For this review, take the finished solid that the model builds, in its own axes (mm). A direction names the side the tool comes from. Round coordinates to 2 decimals unless told otherwise and drop trailing zeros. Order: outer loops, then holes, each group sorted by start corner. A loop starts at its lowest first (then second) coordinate and runs counter-clockwise, first axis right, second up. Notation, with made-up numbers: M -18.5,77 L -0.5,77 A19 ccw -0.5,103 Z; hole C 39,-20.5 d9. An arc over 180 degrees is marked long. Use a Markdown table: item, result.
from build123d import *

# Parameters (mm, degrees)
F0_W     = 11.9395153597
F0_H     = 19.9415329844
F1_DEPTH = 10
F3_DEPTH = 10
F4_W     = 14.7805297747
F4_H     = 20.6165611744
F5_DEPTH = 20


with BuildPart() as f1:
    # F0 (on Top) → F1 (new body)
    with BuildSketch(Plane.XY):
        with BuildLine():
            Line((-31.6270180047, 78.1149193645), (-31.6270180047, 0))
            Line((-31.6270180047, 0), (13.082661666, 0))
            Line((13.082661666, 0), (13.082661666, 19.9415329844))
            Line((13.082661666, 19.9415329844), (25.0221770257, 19.9415329844))
            Line((25.0221770257, 19.9415329844), (25.0221770257, 78.1149193645))
            Line((25.0221770257, 78.1149193645), (0, 78.1149193645))
            Line((0, 78.1149193645), (0, 52.2036328912))
            ThreePointArc((0, 52.2036328912), (-6.414314732, 45.7893181592), (-12.8286294639, 52.2036328912))
            Line((-12.8286294639, 52.2036328912), (-12.8286294639, 78.1149193645))
            Line((-12.8286294639, 78.1149193645), (-31.6270180047, 78.1149193645))
        make_face()
        with Locations((19.0524193458, 9.9707664922)):
            Rectangle(F0_W, F0_H)
    extrude(amount=F1_DEPTH)

    # F2 (on Front) → F3 (join)
    with BuildSketch(Plane.XZ):
        Polygon((-31.6270180047, 0), (25.0221770257, 0), (25.0221770257, 64.1431510448), (-25.0221770257, 64.1431510448), (-31.6270180047, 64.1431510448), align=None)
        with BuildLine():
            Line((-25.0221770257, 64.1431510448), (25.0221770257, 64.1431510448))
            ThreePointArc((25.0221770257, 64.1431510448), (0, 74.3970859516), (-25.0221770257, 64.1431510448))
        make_face()
    extrude(amount=-F3_DEPTH)

    # F4 (on Top) → F5 (cut)
    with BuildSketch(Plane.XY):
        with Locations((17.6329123788, 10.3082805872)):
            Rectangle(F4_W, F4_H)
    extrude(amount=F5_DEPTH, mode=Mode.SUBTRACT)


solid = f1.part
Q1. Add section A-A (y = 66.5). Write out the cut boundary in (x, z).
Determined:
| item | result |
|---|---|
| outline | M -31.63,0 L -12.83,0 L -12.83,10 L -31.63,10 Z; M 0,0 L 25.02,0 L 25.02,10 L 0,10 Z |
Q2. Add section B-B (x = 19.5). Write out the cut boundary in (y, z).
Determined:
| item | result |
|---|---|
| outline | M 0,20 L 10,20 L 10,68.59 L 0,68.59 Z; M 20.62,0 L 78.11,0 L 78.11,10 L 20.62,10 Z |
Q3. Clearance check with flat-ended pins moving along their axes: pin 1 (8 mm diameter, centred on x = -5.5, y = 59, fed in from -Z); pin 2 (6 mm diameter, centred on x = -24.5, y = 41, fed in from +Z); pin 3 (5 mm diameter, centred on x = 20.5, z = 4.5, fed in from -Y); pin 4 (5 mm diameter, centred on x = 20.5, y = 3.5, fed in from -Z). State where each tip first meets the part, or that it passes through.
Determined:
| item | result |
|---|---|
| pin 1 | passes through |
| pin 2 | stops at z = 10 |
| pin 3 | stops at y = 20.62 |
| pin 4 | stops at z = 20 |
Q4. Add section D-D (x = 3). Write out the cut boundary in (y, z).
Determined:
| item | result |
|---|---|
| outline | M 0,0 L 78.11,0 L 78.11,10 L 10,10 L 10,74.27 L 0,74.27 Z |
Q5. Draft analysis for pull direction X (two halves, no side actions). For faces 4 (the flat face through (-12.829, 65, 5)), 5 (the flat face through (10.243, 8, 8)), 6 (the flat face through (18, 5, 20)), 7 (the flat face through (0, 65, 5)), state which applies: pulls with the +X half, pulls with the -X half, needs draft (parallel to the pull), parting line crosses it, or undercut.
Determined:
| item | result |
|---|---|
| face 4 | undercut |
| face 5 | pulls with the +X half |
| face 6 | needs draft |
| face 7 | undercut |
Q6. Wall thickness on line 1 along Y through (x, z) = (-4, 59); line 2 along Z through (x, y) = (-23.5, 5.5): over which ranges is each line inside the solid? List them lowest first. Write a range as [from, to].
Determined:
| item | result |
|---|---|
| line 1 | y = [0, 10] |
| line 2 | z = [0, 65.56] |
Q7. Machinability: for faces 1 (the flat face through (-4, 45, 10)), 2 (the flat face through (18, 20.617, 5)), 3 (the flat face through (-28, 5, 64.143)), which of the approach directions +Z, -Z, +X, -X, +Y, -Y give a long, thin tool a straight path to every point of the face, cutting with its end or side? Answer none if there is none.
Determined:
| item | result |
|---|---|
| face 1 | +Z, +X, -X, +Y |
| face 2 | +Z, -Z, +X, -Y |
| face 3 | +Z, -X, +Y, -Y |
Q8. Add section C-C (z = 5.5). Write out the cut boundary in (x, y).
Determined:
| item | result |
|---|---|
| outline | M -31.63,0 L 10.24,0 L 10.24,20.62 L 25.02,20.62 L 25.02,78.11 L 0,78.11 L 0,52.2 A6.41 cw -12.83,52.2 L -12.83,78.11 L -31.63,78.11 Z |
